Study the drawing (mm; zero at the part's minimum x, y, z) and answer. A direction names the side the tool comes from. Give positions to 0.01 mm unless a question says otherwise; leave off trailing zeros. Loops run counter-clockwise (first coordinate to the right, second up) from the corner with the lowest first, then second, coordinate; pieces in that order, holes last. Notation, with made-up numbers: (76, 88) - (105, 88) arc R9 cw to (105, 95) - close; hole circle Ø11 at (-21.5, 52). An arc over 180 degrees is marked (long way). One line per item, written item: value. Start each with the question number.
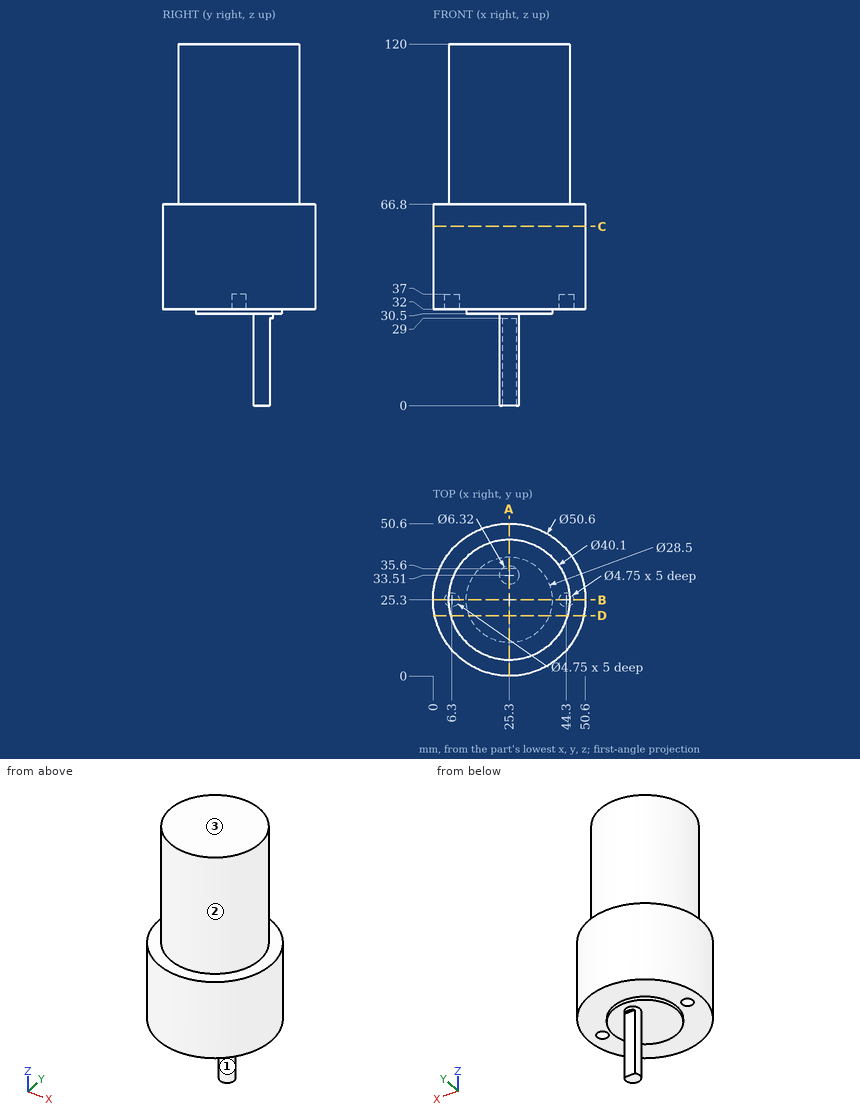
1. Flat-ended cylindrical pins translate along their axes: pin 1 (1.5 mm diameter, centred on x = 27, y = 15, fed in from -Z); pin 2 (5 mm diameter, centred on x = 26, z = 17.5, fed in from +Y); pin 3 (0.5 mm diameter, centred on x = 26.5, y = 36, fed in from -Z). Find the tip coordinate at first contact, or state that the pin passes through.
2. A cutting plane is placed at B-B (y = 25.3). Determine the outline of the cut face in (x, z) (3 decimals).
3. A cutting plane is placed at A-A (x = 25.3). Determine the outline of the cut face in (y, z).
4. For the marked faces 1, 2 and 3, determine the directions among +Z, -Z, +X, -X, +Y, -Y from which every point of the face is accessible in a straight line to the end or side of a thin tool.
5. Find the intervals of material crossed by L1, parallel to Z at x = 26.5, y = 8; L2, parallel to Y at x = 44.3, z = 33.6 (3 decimals); L3, parallel to Z at x = 44.5, y = 11, in increasing order. Write a range as [from, to].
6. A cutting plane is placed at C-C (z = 59.5). Determine the outline of the cut face in (x, y), plus the area to 3 significant figures.
7. A cutting plane is placed at D-D (y = 20). Determine the outline of the cut face in (x, z).
Results below:
1. pin 1: stops at z = 30.5
1. pin 2: stops at y = 35.6
1. pin 3: stops at z = 29
2. outline: (0, 32) - (3.925, 32) - (3.925, 37) - (8.675, 37) - (8.675, 32) - (11.05, 32) - (11.05, 30.5) - (39.55, 30.5) - (39.55, 32) - (41.925, 32) - (41.925, 37) - (46.675, 37) - (46.675, 32) - (50.6, 32) - (50.6, 66.8) - (45.35, 66.8) - (45.35, 120) - (5.25, 120) - (5.25, 66.8) - (0, 66.8) - close
3. outline: (0, 32) - (11.05, 32) - (11.05, 30.5) - (30.35, 30.5) - (30.35, 0) - (35.6, 0) - (35.6, 29) - (36.67, 29) - (36.67, 30.5) - (39.55, 30.5) - (39.55, 32) - (50.6, 32) - (50.6, 66.8) - (45.35, 66.8) - (45.35, 120) - (5.25, 120) - (5.25, 66.8) - (0, 66.8) - close
4. face 1: -Z
4. face 2: +Z
4. face 3: +Z, +X, -X, +Y, -Y
5. L1: z = [32, 120]
5. L2: y = [8.594, 22.925], [27.675, 42.006]
5. L3: z = [32, 66.8]
6. outline: circle Ø50.6 at (25.3, 25.3)
6. area: 2,010 mm^2
7. outline: (0.56, 32) - (12.07, 32) - (12.07, 30.5) - (38.53, 30.5) - (38.53, 32) - (50.04, 32) - (50.04, 66.8) - (44.64, 66.8) - (44.64, 120) - (5.96, 120) - (5.96, 66.8) - (0.56, 66.8) - close
